```python
from build123d import *

# Parameters (mm, degrees)
F0_W         = 76.2
F0_H         = 76.2
F1_DEPTH     = 76.2
F2_T         = -2.54
F3_T1_DEPTH  = 83.82
F3_T3_DEPTH  = 83.82
F3_T5_DEPTH  = 83.82
F3_T7_DEPTH  = 101.6
F3_T9_DEPTH  = 101.6
F3_S13_W     = 5.08
F3_S13_H     = 5.08
F3_T14_DEPTH = 5.08


# Not quite as in the source:
# - a fillet or chamfer that OpenCascade refuses, or shapes differently, is made with other operations: its cross-section is extruded or revolved along the edge and cut away or added


with BuildPart() as f1:
    # F0 (on Front) → F1 (new body)
    with BuildSketch(Plane.XZ):
        with Locations((-1.2479908764, -6.1416627283)):
            Rectangle(F0_W, F0_H)
    extrude(amount=F1_DEPTH)

    # F2
    f2_openings = [f1.faces().sort_by_distance(p)[0] for p in [
        (-1.247991, 0, -6.141663),
    ]]
    offset(amount=F2_T, openings=f2_openings)

    # F3: fillet of radius 5.08 on 5 edges, made by hand

    # F3_s2 → F3_t1 (cut)
    with BuildSketch(Plane.XY.offset(-39.1616627283)):
        with BuildLine():
            ThreePointArc((36.8520091236, -71.12), (35.364111572, -74.7121024484), (31.7720091236, -76.2))
            Line((31.7720091236, -76.2), (36.8520091236, -76.2))
            Line((36.8520091236, -76.2), (36.8520091236, -71.12))
        make_face()
    extrude(amount=F3_T1_DEPTH, mode=Mode.SUBTRACT)

    # F3_s4 → F3_t3 (cut)
    with BuildSketch(Plane.YZ.offset(-52.0479908764)):
        with BuildLine():
            ThreePointArc((-71.12, -44.2416627283), (-74.7121024484, -42.7537651767), (-76.2, -39.1616627283))
            Line((-76.2, -39.1616627283), (-76.2, -44.2416627283))
            Line((-76.2, -44.2416627283), (-71.12, -44.2416627283))
        make_face()
    extrude(amount=F3_T3_DEPTH, mode=Mode.SUBTRACT)

    # F3_s6 → F3_t5 (cut)
    with BuildSketch(Plane.XZ.offset(-12.7)):
        with BuildLine():
            ThreePointArc((31.7720091236, -44.2416627283), (35.364111572, -42.7537651767), (36.8520091236, -39.1616627283))
            Line((36.8520091236, -39.1616627283), (36.8520091236, -44.2416627283))
            Line((36.8520091236, -44.2416627283), (31.7720091236, -44.2416627283))
        make_face()
    extrude(amount=F3_T5_DEPTH, mode=Mode.SUBTRACT)

    # F3_s8 → F3_t7 (cut)
    with BuildSketch(Plane.XY.offset(-56.9416627283)):
        with BuildLine():
            ThreePointArc((36.8520091236, -5.08), (35.364111572, -1.4878975516), (31.7720091236, 0))
            Line((31.7720091236, 0), (36.8520091236, 0))
            Line((36.8520091236, 0), (36.8520091236, -5.08))
        make_face()
    extrude(amount=F3_T7_DEPTH, mode=Mode.SUBTRACT)

    # F3_s10 → F3_t9 (cut)
    with BuildSketch(Plane.XZ.offset(-12.7)):
        with BuildLine():
            ThreePointArc((31.7720091236, 31.9583372717), (35.364111572, 30.4704397201), (36.8520091236, 26.8783372717))
            Line((36.8520091236, 26.8783372717), (36.8520091236, 31.9583372717))
            Line((36.8520091236, 31.9583372717), (31.7720091236, 31.9583372717))
        make_face()
    extrude(amount=F3_T9_DEPTH, mode=Mode.SUBTRACT)


with BuildPart() as f3_tool12:
    # F3_s13 → F3_t14 (new body)
    with BuildSketch(Plane.XY.offset(-39.1616627283)):
        with Locations((34.3120091236, -73.66)):
            Rectangle(F3_S13_W, F3_S13_H)
    extrude(amount=-F3_T14_DEPTH)

    # F3_s15 → F3_t16 (revolve, cut)
    with BuildSketch(Plane(origin=(31.7720091236, -71.12, -39.1616627283), x_dir=(-0.7071067812, 0.7071067812, 0), z_dir=(-0.7071067812, -0.7071067812, 0))):
        with BuildLine():
            ThreePointArc((0, -5.08), (5.08, 0), (0, 5.08))
            Line((0, 5.08), (0, -5.08))
        make_face()
    revolve(axis=Axis((31.7720091236, -71.12, -39.1616627283), (0, 0, -1)), mode=Mode.SUBTRACT)


with BuildPart() as f1_1:
    add(f1.part)

    # F3_t11: cut F3_tool12
    add(f3_tool12.part, mode=Mode.SUBTRACT)


solid = f1_1.part
```
Can you work these out from the model? Positions are in its coordinate system, mm. A direction names the side the tool comes from. Give positions to 0.01 mm unless a question says otherwise; leave off trailing zeros. Order: outer loops, then holes, each group sorted by start corner. A loop starts at its lowest first (then second) coordinate and runs counter-clockwise, first axis right, second up. Notation, with made-up numbers: M -23.5,37.5 L 14.5,37.5 A30 ccw 14.5,72.5 Z; hole C 30.25,26.5 d5. An arc over 180 degrees is marked long. One line per item, written item: value.
1) On a 3-axis mill with a long thin cutter (end or side, diameter ignored), from which of +Z, -Z, +X, -X, +Y, -Y can I reach the whole of each face in a straight line? I mean faces 4 (the face through (-36.808, -36, -7)), 5 (the face through (-39.348, -38, -7)). Say none if no direction works.
Answer sheet:
face 4: +Y
face 5: +Z, -Z, -X, +Y, -Y
2) For P1, Ø4, axis at x = 27, z = 21, coming from the +Y side, with a flat end and sliding along its axis, tell me the tip position at first contact or that it passes through.
Answer sheet:
P1: stops at y = -73.66
3) Please list where these lines run through material, in increasing order: line 1 along Z through (x, y) = (1, -65); line 2 along X through (y, z) = (-65.5, -0.5); line 3 along X through (y, z) = (-71.5, 1).
Answer sheet:
line 1: z = -44.24 to -41.7, 29.42 to 31.96
line 2: x = -39.35 to -36.81, 34.31 to 36.85
line 3: x = -39.35 to -36.81, 34.31 to 36.84
4) I want a section at C-C, the plane x = -1.5. List the corners of the cut face in (y, z) for me, plus the area to 3 significant figures.
Answer sheet:
outline: M -76.2,-39.16 A5.08 ccw -71.12,-44.24 L 0,-44.24 L 0,-41.7 L -73.66,-41.7 L -73.66,29.42 L 0,29.42 L 0,31.96 L -76.2,31.96 Z
area: 562 mm^2
5) I want a section at B-B, the plane z = -30. List the corners of the cut face in (x, y) for me, plus the area to 3 significant figures.
Answer sheet:
outline: M -39.35,-76.2 L 31.77,-76.2 A5.08 ccw 36.85,-71.12 L 36.85,-5.08 A5.08 ccw 34.31,-0.68 L 34.31,-73.66 L -36.81,-73.66 L -36.81,0 L -39.35,0 Z
area: 557 mm^2
6) We'd pull the mould along X, two halves only. Please class faces 1 (the face through (35.965, -2.212, -6.675)), 2 (the face through (-2, -36, -41.702)), 3 (the face through (-4.286, -74.672, -42.793)): released by +X, released by -X, zero draft, split by the parting line, or undercut.
Answer sheet:
face 1: released by +X
face 2: undercut
face 3: zero draft
7) I want a section at A-A, the plane y = -29. List the corners of the cut face in (x, z) for me.
Answer sheet:
outline: M -39.35,-44.24 L 31.77,-44.24 A5.08 ccw 36.85,-39.16 L 36.85,26.88 A5.08 ccw 31.77,31.96 L -39.35,31.96 Z; hole M -36.81,-41.7 L 34.31,-41.7 L 34.31,29.42 L -36.81,29.42 Z
